```python
from build123d import *

# Parameters (mm, degrees)
SKETCH2_R           = 1.6
SKETCH2_R_2         = 3.5
BOSS_EXTRUDE1_DEPTH = 1.75
SKETCH3_R           = 3
CUT_EXTRUDE2_DEPTH  = 0.3
CHAMFER1_SIZE       = 1.4


with BuildPart() as part:
    # Sketch2 → Boss-Extrude1 (new body)
    # profile 1 of 4: a face of its own
    with BuildSketch(Plane(origin=(277.94406545, -368.782269, 0), x_dir=(0.99993266408239, 0.011604624125499034, 0), z_dir=(0, 0, 1))):
        with BuildLine():
            Line((-273.645770216, 387.793792834), (-273.645770216, 371.982873115))
            Line((-273.645770216, 371.982873115), (-270.995770216, 371.982873115))
            Line((-270.995770216, 371.982873115), (-270.995770216, 373.982873115))
            Line((-270.995770216, 373.982873115), (-271.645770216, 373.982873115))
            ThreePointArc((-271.645770216, 373.982873115), (-272.352876997, 374.275766334), (-272.645770216, 374.982873115))
            Line((-272.645770216, 374.982873115), (-272.645770216, 375.582873115))
            ThreePointArc((-272.645770216, 375.582873115), (-272.352876997, 376.289979896), (-271.645770216, 376.582873115))
            Line((-271.645770216, 376.582873115), (-267.145770216, 376.582873115))
            ThreePointArc((-267.145770216, 376.582873115), (-266.438663434, 376.289979896), (-266.145770216, 375.582873115))
            Line((-266.145770216, 375.582873115), (-266.145770216, 374.982873115))
            ThreePointArc((-266.145770216, 374.982873115), (-266.438663434, 374.275766334), (-267.145770216, 373.982873115))
            Line((-267.145770216, 373.982873115), (-267.795770216, 373.982873115))
            Line((-267.795770216, 373.982873115), (-267.795770216, 371.982873115))
            Line((-267.795770216, 371.982873115), (-240.495770216, 371.982873115))
            Line((-240.495770216, 371.982873115), (-240.495770216, 373.982873115))
            Line((-240.495770216, 373.982873115), (-241.145770216, 373.982873115))
            ThreePointArc((-241.145770216, 373.982873115), (-241.852876997, 374.275766334), (-242.145770216, 374.982873115))
            Line((-242.145770216, 374.982873115), (-242.145770216, 375.582873115))
            ThreePointArc((-242.145770216, 375.582873115), (-241.852876997, 376.289979896), (-241.145770216, 376.582873115))
            Line((-241.145770216, 376.582873115), (-236.645770216, 376.582873115))
            ThreePointArc((-236.645770216, 376.582873115), (-235.938663434, 376.289979896), (-235.645770216, 375.582873115))
            Line((-235.645770216, 375.582873115), (-235.645770216, 374.982873115))
            ThreePointArc((-235.645770216, 374.982873115), (-235.938663434, 374.275766334), (-236.645770216, 373.982873115))
            Line((-236.645770216, 373.982873115), (-237.295770216, 373.982873115))
            Line((-237.295770216, 373.982873115), (-237.295770216, 371.982873115))
            Line((-237.295770216, 371.982873115), (-231.145770216, 371.982873115))
            Line((-231.145770216, 371.982873115), (-231.145770216, 391.107179671))
            ThreePointArc((-231.145770216, 391.107179671), (-238.062806241, 390.349641022), (-231.473692961, 392.586343587))
            Line((-231.473692961, 392.586343587), (-236.545112102, 403.462037031))
            ThreePointArc((-236.545112102, 403.462037031), (-236.300153332, 402.740411764), (-236.217189356, 401.982873115))
            ThreePointArc((-236.217189356, 401.982873115), (-238.959651202, 398.565836981), (-242.889267039, 400.503710116))
            ThreePointArc((-242.889267039, 400.503710116), (-243.006113356, 403.179944092), (-241.196353273, 405.15495037))
            Line((-241.196353273, 405.15495037), (-271.624933816, 390.965870235))
            ThreePointArc((-271.624933816, 390.965870235), (-268.26522144, 390.745662801), (-266.645770216, 387.793792834))
            ThreePointArc((-266.645770216, 387.793792834), (-270.145770216, 384.293792834), (-273.645770216, 387.793792834))
        make_face()
        with Locations(Location((-242.145770216, 386.482873115, 0), (0, 0, 359.335089091))):
            Circle(SKETCH2_R, mode=Mode.SUBTRACT)
        with Locations(Location((-264.6406535, 390.360870917, 0), (0, 0, 359.335089091))):
            Circle(SKETCH2_R, mode=Mode.SUBTRACT)
        with BuildLine():
            Line((-242.994921177, 400.730286146), (-242.889267039, 400.503710116))
            Line((-242.889267039, 400.503710116), (-242.783612046, 400.277132252))
            ThreePointArc((-242.783612046, 400.277132252), (-242.750227212, 399.512493847), (-243.267301571, 398.948206203))
            Line((-243.267301571, 398.948206203), (-260.033995631, 391.129768361))
            ThreePointArc((-260.033995631, 391.129768361), (-260.798634036, 391.096383528), (-261.36292168, 391.613457887))
            Line((-261.36292168, 391.613457887), (-261.574230811, 392.06661178))
            ThreePointArc((-261.574230811, 392.06661178), (-261.607615645, 392.831250185), (-261.090541285, 393.395537829))
            Line((-261.090541285, 393.395537829), (-244.323847225, 401.213975671))
            ThreePointArc((-244.323847225, 401.213975671), (-243.55920882, 401.247360505), (-242.994921177, 400.730286146))
        make_face(mode=Mode.SUBTRACT)
    # profile 2 of 4: a face of its own
    with BuildSketch(Plane(origin=(277.94406545, -368.782269, 0), x_dir=(0.99993266408239, 0.011604624125499034, 0), z_dir=(0, 0, 1))):
        with Locations((-270.145770216, 387.793792834)):
            Circle(SKETCH2_R_2)
    # profile 3 of 4: a face of its own
    with BuildSketch(Plane(origin=(277.94406545, -368.782269, 0), x_dir=(0.99993266408239, 0.011604624125499034, 0), z_dir=(0, 0, 1))):
        with Locations((-234.645770216, 391.107179671)):
            Circle(SKETCH2_R_2)
    # profile 4 of 4: a face of its own
    with BuildSketch(Plane(origin=(277.94406545, -368.782269, 0), x_dir=(0.99993266408239, 0.011604624125499034, 0), z_dir=(0, 0, 1))):
        with Locations((-239.717189356, 401.982873115)):
            Circle(SKETCH2_R_2)
        with Locations(Location((-239.717189356, 401.982873115, 0), (0, 0, 359.335089091))):
            Circle(SKETCH2_R, mode=Mode.SUBTRACT)
    extrude(amount=BOSS_EXTRUDE1_DEPTH)

    # Sketch3 → Cut-Extrude2 (cut)
    with BuildSketch(Plane.XY.offset(1.75)):
        with Locations((8.791240591, 18.481261297)):
            Circle(SKETCH3_R)
        with Locations((31.329611869, 14.864569289)):
            Circle(SKETCH3_R)
        with Locations((33.578157523, 30.39170835)):
            Circle(SKETCH3_R)
    extrude(amount=-CUT_EXTRUDE2_DEPTH, mode=Mode.SUBTRACT)

    # Chamfer1
    chamfer1_edges = [part.edges().sort_by_distance(p)[0] for p in [
        (7.191240591, 18.481261297, 1.45),
        (29.729611869, 14.864569289, 1.45),
        (31.978157523, 30.39170835, 1.45),
    ]]
    chamfer(chamfer1_edges, length=CHAMFER1_SIZE - 0.0001)  # a hair under: the kernel refuses the full size


solid = part.part
```
Verification items for the finished model (mm, model axes). A direction names the side the tool comes from. Coordinates: 2 decimals unless noted, no trailing zeros. Loops run counter-clockwise (first coordinate to the right, second up) from the corner with the lowest first, then second, coordinate; pieces in that order, holes last. Notation, with made-up numbers: (-16.5, 70) - (28.5, 70) arc R18 cw to (28.5, 75) - close; hole circle Ø9 at (26, 50). An arc over 180 degrees is marked (long way). Return JSON: item names as keys, results as strings.
1. Mould release check, pull along X, two halves, no side actions. Record for faces 1 (the cylindrical face through (37.65, 4.75, 0.86)), 2 (the cylindrical face through (37.69, 2.74, 0.86)), 3 (the flat face through (21, 14, 1.75)), 4 (the cylindrical face through (34.773, 33.681, 0.863)): +X half, -X half, draft (parallel to the pull), parting line (faces both ways), or undercut.
Established:
{"face 1": "undercut", "face 2": "undercut", "face 3": "draft", "face 4": "parting line"}
2. Section check D-D, the plane x = 40. Record the boundary of the cut face in (y, z).
Established:
{"outline": "(0.46, 0) - (25.11, 0) - (25.11, 1.75) - (0.46, 1.75) - close"}
3. Section check C-C, the plane x = 4. Record the boundary of the cut face in (y, z), then the cut area to 3 significant figures.
Established:
{"outline": "(4.65, 0) - (20.06, 0) - (20.06, 1.75) - (4.65, 1.75) - close", "area": "27.0 mm2"}
4. Section check B-B, the plane y = 24.5. Record the boundary of the cut face in (x, z), then the cut area to 3 significant figures.
Established:
{"outline": "(13.24, 0) - (18.43, 0) - (18.43, 1.75) - (13.24, 1.75) - close; (24.2, 0) - (40.29, 0) - (40.29, 1.75) - (24.2, 1.75) - close", "area": "37.2 mm2"}
5. Thickness scan on L1, parallel to Y at x = 32, z = 1.6; L2, parallel to X at y = 21, z = 1.5; L3, parallel to X at y = 28.5, z = 0.95. Record the ranges inside material, lowest first.
Established:
{"L1": "y = 0.37 to 2.49, 4.87 to 11.94, 17.79 to 27.84, 32.94 to 33.52", "L2": "x = 5.95 to 7.16, 10.42 to 11.8, 16.92 to 41.97", "L3": "x = 21.56 to 26.76, 30.59 to 31.94, 35.21 to 38.37"}
6. Tool access check on faces 5 (the cylindrical face through (12.63, 19.26, 0.86)), 6 (the cylindrical face through (31.37, 32.42, 1.6)), 7 (the flat face through (21, 14, 0)). Record the directions out of +Z, -Z, +X, -X, +Y, -Y that give a thin tool (end or side, any length) a straight path to the whole face; none if there is none.
Established:
{"face 5": "+Z, -Z", "face 6": "+Z", "face 7": "-Z, +X, -X, +Y, -Y"}
7. Go/stop test with flat-tipped pins: pin 1 (8 mm diameter, centred on x = 33.58, y = 30.39, fed in from +Z); pin 2 (1 mm diameter, centred on y = 12.5, z = 0.5, fed in from +X); pin 3 (5 mm diameter, centred on x = 8.79, y = 18.48, fed in from +Z); pin 4 (1.8 mm diameter, centred on x = 9, y = 17.5, fed in from +Z). Record where each tip stops, or that it passes through.
Established:
{"pin 1": "stops at z = 1.75", "pin 2": "stops at x = 42.36", "pin 3": "stops at z = 0.95", "pin 4": "stops at z = 0.35"}
8. Section check A-A, the plane x = 26. Record the boundary of the cut face in (y, z).
Established:
{"outline": "(0.3, 0) - (25.36, 0) - (25.36, 1.75) - (0.3, 1.75) - close; (28.14, 0) - (30.63, 0) - (30.63, 1.75) - (28.14, 1.75) - close"}
